Design review of the part built by this model. Coordinates are the model's own, in mm. Face numbers are marked on the shaded views. A direction names the side the tool comes from. Give positions to 0.01 mm unless a question says otherwise; leave off trailing zeros. Write each loop counter-clockwise with the first axis right and the second up, starting at its lowest first coordinate (ties: lowest second). Pieces come first, ordered by that corner, then holes. Notation, with made-up numbers: (-32, 68.25) -> (0, 68.25) arc R20 ccw to (0, 93.25) -> close; hole circle Ø11 at (-38.5, 69.5). An arc over 180 degrees is marked (long way). Answer as a JSON object with one key per item and string values.
```python
from build123d import *

# Parameters (mm, degrees)
SKETCH1_W                                      = 135
SKETCH1_H                                      = 103
BOSS_EXTRUDE1_DEPTH                            = 13
SKETCH2_W                                      = 127.02
SKETCH2_H                                      = 95.02
CUT_EXTRUDE1_DEPTH                             = 10
SKETCH3_R                                      = 6
CUT_EXTRUDE2_DEPTH                             = 2
FILLET1_R                                      = 1
FILLET1_OF_MIRROR1_R                           = 1
SKETCH4_R                                      = 6
CUT_EXTRUDE3_DEPTH                             = 2
FILLET2_R                                      = 1
FILLET2_OF_MIRROR2_R                           = 1
SKETCH5_W                                      = 31
SKETCH5_H                                      = 2.5
CUT_EXTRUDE4_DEPTH                             = 5
SKETCH6_W                                      = 135
SKETCH6_H                                      = 103
CUT_EXTRUDE5_DEPTH                             = 3.5
SKETCH7_W                                      = 33
SKETCH7_H                                      = 12
CUT_EXTRUDE6_DEPTH                             = 5
SKETCH8_OUTSIDE_W                              = 171.014
SKETCH8_OUTSIDE_H                              = 139.014
SKETCH8_OUTSIDE_W_2                            = 131
SKETCH8_OUTSIDE_H_2                            = 99
CUT_AROUND_SIDE_FOR_FRICTION_FITTING_COV_DEPTH = 1.5
SKETCH9_W                                      = 15
SKETCH9_H                                      = 2
CUT_EXTRUDE8_DEPTH                             = 1.5
FILLET3_R                                      = 5
FILLET4_R                                      = 2
SKETCH14_W                                     = 8.2
SKETCH14_H                                     = 1.5
CUT_EXTRUDE13_DEPTH                            = 4
SKETCH16_W                                     = 8.2
SKETCH16_H                                     = 1.5
CUT_EXTRUDE14_DEPTH                            = 4
SKETCH17_W                                     = 1.99
SKETCH17_H                                     = 1.5
CUT_EXTRUDE15_DEPTH                            = 9.3
CUT_EXTRUDE15_DEPTH_BACK                       = 1.1
SKETCH18_W                                     = 1.99
SKETCH18_H                                     = 1.5
CUT_EXTRUDE16_DEPTH                            = 9.3
CUT_EXTRUDE16_DEPTH_BACK                       = 1.1
SKETCH19_W                                     = 10.4
SKETCH19_H                                     = 4.692472087
SKETCH19_W_2                                   = 10.469305177
SKETCH19_H_2                                   = 5.245813632
CUT_EXTRUDE17_DEPTH                            = 3.1
SKETCH23_W                                     = 3.99
SKETCH23_H                                     = 3.1
BOSS_EXTRUDE2_DEPTH                            = 0.069305
CUT_EXTRUDE20_DEPTH                            = 0.2
CUT_EXTRUDE21_DEPTH                            = 0.4
CUT_EXTRUDE22_DEPTH                            = 0.3
CUT_EXTRUDE23_DEPTH                            = 0.3
SCALE1_SCALE                                   = 1.015


with BuildPart() as part:
    # Sketch1 → Boss-Extrude1 (new body)
    with BuildSketch(Plane(origin=(0, 0, 0), x_dir=(1, 0, 0), z_dir=(0, 1, 0))):
        Rectangle(SKETCH1_W, SKETCH1_H)
    extrude(amount=BOSS_EXTRUDE1_DEPTH)

    # Sketch2 → Cut-Extrude1 (cut)
    with BuildSketch(Plane(origin=(0, 13, 0), x_dir=(1, 0, 0), z_dir=(0, 1, 0))):
        Rectangle(SKETCH2_W, SKETCH2_H)
    extrude(amount=-CUT_EXTRUDE1_DEPTH, mode=Mode.SUBTRACT)

    # Sketch3 → Cut-Extrude2 (cut)
    with BuildSketch(Plane(origin=(0, 3, 0), x_dir=(1, 0, 0), z_dir=(0, 1, 0))):
        with Locations((-52.51, -36.51)):
            Circle(SKETCH3_R)
    cut_extrude2 = extrude(amount=-CUT_EXTRUDE2_DEPTH, mode=Mode.SUBTRACT)

    # Fillet1
    fillet1_edges = [part.edges().sort_by_distance(p)[0] for p in [
        (-58.51, 1, 36.51),
    ]]
    fillet(fillet1_edges, radius=FILLET1_R)

    # Mirror1: Cut-Extrude2 across plane
    add(cut_extrude2.mirror(Plane(origin=(0, 0, 0), x_dir=(0, 0, 1), z_dir=(1, 0, 0))), mode=Mode.SUBTRACT)

    # Fillet1 of Mirror1
    fillet1_of_mirror1_edges = [part.edges().sort_by_distance(p)[0] for p in [
        (58.51, 1, 36.51),
    ]]
    fillet(fillet1_of_mirror1_edges, radius=FILLET1_OF_MIRROR1_R)

    # Sketch4 → Cut-Extrude3 (cut)
    with BuildSketch(Plane(origin=(0, 3, 0), x_dir=(1, 0, 0), z_dir=(0, 1, 0))):
        with Locations((-44.51, 36.51)):
            Circle(SKETCH4_R)
    cut_extrude3 = extrude(amount=-CUT_EXTRUDE3_DEPTH, mode=Mode.SUBTRACT)

    # Fillet2
    fillet2_edges = [part.edges().sort_by_distance(p)[0] for p in [
        (-50.51, 1, -36.51),
    ]]
    fillet(fillet2_edges, radius=FILLET2_R)

    # Mirror2: Cut-Extrude3 across plane
    add(cut_extrude3.mirror(Plane(origin=(0, 0, 0), x_dir=(0, 0, 1), z_dir=(1, 0, 0))), mode=Mode.SUBTRACT)

    # Fillet2 of Mirror2
    fillet2_of_mirror2_edges = [part.edges().sort_by_distance(p)[0] for p in [
        (50.51, 1, -36.51),
    ]]
    fillet(fillet2_of_mirror2_edges, radius=FILLET2_OF_MIRROR2_R)

    # Sketch5 → Cut-Extrude4 (cut)
    with BuildSketch(Plane.ZY.offset(67.5)):
        with Locations((-30.05, 9.25)):
            Rectangle(SKETCH5_W, SKETCH5_H)
    extrude(amount=-CUT_EXTRUDE4_DEPTH, mode=Mode.SUBTRACT)

    # Sketch6 → Cut-Extrude5 (cut)
    with BuildSketch(Plane(origin=(0, 13, 0), x_dir=(1, 0, 0), z_dir=(0, 1, 0))):
        Rectangle(SKETCH6_W, SKETCH6_H)
    extrude(amount=-CUT_EXTRUDE5_DEPTH, mode=Mode.SUBTRACT)

    # Sketch7 → Cut-Extrude6 (cut)
    with BuildSketch(Plane(origin=(67.5, 0, 0), x_dir=(0, 0, -1), z_dir=(1, 0, 0))):
        with Locations((-3, 14)):
            Rectangle(SKETCH7_W, SKETCH7_H)
    extrude(amount=-CUT_EXTRUDE6_DEPTH, mode=Mode.SUBTRACT)

    # Sketch8 outside → Cut Around side for friction fitting cover (cut)
    with BuildSketch(Plane(origin=(0, 9.5, 0), x_dir=(1, 0, 0), z_dir=(0, 1, 0))):
        Rectangle(SKETCH8_OUTSIDE_W, SKETCH8_OUTSIDE_H)
        Rectangle(SKETCH8_OUTSIDE_W_2, SKETCH8_OUTSIDE_H_2, mode=Mode.SUBTRACT)
    extrude(amount=-CUT_AROUND_SIDE_FOR_FRICTION_FITTING_COV_DEPTH, mode=Mode.SUBTRACT)

    # Sketch9 → Cut-Extrude8 (cut)
    with BuildSketch(Plane(origin=(0, 8, 0), x_dir=(1, 0, 0), z_dir=(0, 1, 0))):
        with Locations((0, -50.5)):
            Rectangle(SKETCH9_W, SKETCH9_H)
    extrude(amount=-CUT_EXTRUDE8_DEPTH, mode=Mode.SUBTRACT)

    # Fillet3
    fillet3_edges = [part.edges().sort_by_distance(p)[0] for p in [
        (67.5, 4, 51.5),
        (-67.5, 4, 51.5),
        (-67.5, 4, -51.5),
        (67.5, 4, -51.5),
    ]]
    fillet(fillet3_edges, radius=FILLET3_R)

    # Fillet4
    fillet4_edges = [part.edges().sort_by_distance(p)[0] for p in [
        (67.5, 0, 0),
        (0, 0, 51.5),
        (-67.5, 0, 0),
        (0, 0, -51.5),
        (-66.035533906, 0, 50.035533906),
        (-66.035533906, 0, -50.035533906),
        (66.035533906, 0, -50.035533906),
        (66.035533906, 0, 50.035533906),
    ]]
    fillet(fillet4_edges, radius=FILLET4_R)

    # Sketch14 → Cut-Extrude13 (cut)
    with BuildSketch(Plane.XY.offset(49.5)):
        with Locations((-56.5, 8.75)):
            Rectangle(SKETCH14_W, SKETCH14_H)
    extrude(amount=-CUT_EXTRUDE13_DEPTH, mode=Mode.SUBTRACT)

    # Sketch16 → Cut-Extrude14 (cut)
    with BuildSketch(Plane.XY.offset(49.5)):
        with Locations((-41.5, 8.75)):
            Rectangle(SKETCH16_W, SKETCH16_H)
    extrude(amount=-CUT_EXTRUDE14_DEPTH, mode=Mode.SUBTRACT)

    # Sketch17 → Cut-Extrude15 (cut, two sides)
    with BuildSketch(Plane(origin=(-60.6, 0, 0), x_dir=(0, 0, -1), z_dir=(1, 0, 0))) as cut_extrude15_sk:
        with Locations((-48.505, 8.75)):
            Rectangle(SKETCH17_W, SKETCH17_H)
    extrude(amount=CUT_EXTRUDE15_DEPTH, mode=Mode.SUBTRACT)
    extrude(cut_extrude15_sk.sketch, amount=-CUT_EXTRUDE15_DEPTH_BACK, mode=Mode.SUBTRACT)

    # Sketch18 → Cut-Extrude16 (cut, two sides)
    with BuildSketch(Plane(origin=(-45.6, 0, 0), x_dir=(0, 0, -1), z_dir=(1, 0, 0))) as cut_extrude16_sk:
        with Locations((-48.505, 8.75)):
            Rectangle(SKETCH18_W, SKETCH18_H)
    extrude(amount=CUT_EXTRUDE16_DEPTH, mode=Mode.SUBTRACT)
    extrude(cut_extrude16_sk.sketch, amount=-CUT_EXTRUDE16_DEPTH_BACK, mode=Mode.SUBTRACT)

    # Sketch19 → Cut-Extrude17 (cut)
    with BuildSketch(Plane(origin=(0, 8, 0), x_dir=(1, 0, 0), z_dir=(0, 1, 0))):
        with Locations((-56.5, -49.856236044)):
            Rectangle(SKETCH19_W, SKETCH19_H)
        with Locations((-41.465347412, -50.132906816)):
            Rectangle(SKETCH19_W_2, SKETCH19_H_2)
    extrude(amount=-CUT_EXTRUDE17_DEPTH, mode=Mode.SUBTRACT)

    # Sketch23 → Boss-Extrude2 (add)
    with BuildSketch(Plane.ZY.offset(36.230694823)):
        with Locations((49.505, 6.45)):
            Rectangle(SKETCH23_W, SKETCH23_H)
    extrude(amount=BOSS_EXTRUDE2_DEPTH)

    # Sketch24 → Cut-Extrude20 (cut)
    with BuildSketch(Plane.ZY.offset(36.3)):
        Polygon((47.51, 4.9), (47.51, 9.5), (49.5, 9.5), (49.5, 8), (51.5, 8), (51.5, 4.9), align=None)
    extrude(amount=-CUT_EXTRUDE20_DEPTH, mode=Mode.SUBTRACT)

    # Sketch25 → Cut-Extrude21 (cut)
    with BuildSketch(Plane(origin=(-46.7, 0, 0), x_dir=(0, 0, -1), z_dir=(1, 0, 0))):
        Polygon((-51.5, 4.9), (-47.51, 4.9), (-47.51, 9.5), (-49.5, 9.5), (-49.5, 8), (-51.5, 8), align=None)
    extrude(amount=-CUT_EXTRUDE21_DEPTH, mode=Mode.SUBTRACT)

    # Sketch26 → Cut-Extrude22 (cut)
    with BuildSketch(Plane.ZY.offset(51.3)):
        Polygon((47.51, 9.5), (47.51, 4.9), (51.5, 4.9), (51.5, 8), (49.5, 8), (49.5, 9.5), align=None)
    extrude(amount=-CUT_EXTRUDE22_DEPTH, mode=Mode.SUBTRACT)

    # Sketch27 → Cut-Extrude23 (cut)
    with BuildSketch(Plane(origin=(-61.7, 0, 0), x_dir=(0, 0, -1), z_dir=(1, 0, 0))):
        Polygon((-51.5, 4.9), (-47.51, 4.9), (-47.51, 9.5), (-49.5, 9.5), (-49.5, 8), (-51.5, 8), align=None)
    extrude(amount=-CUT_EXTRUDE23_DEPTH, mode=Mode.SUBTRACT)


with BuildPart() as part_1:
    # Scale1: scaled about (0, 0, 0)
    add(part.part.scale(SCALE1_SCALE))


solid = part_1.part
```
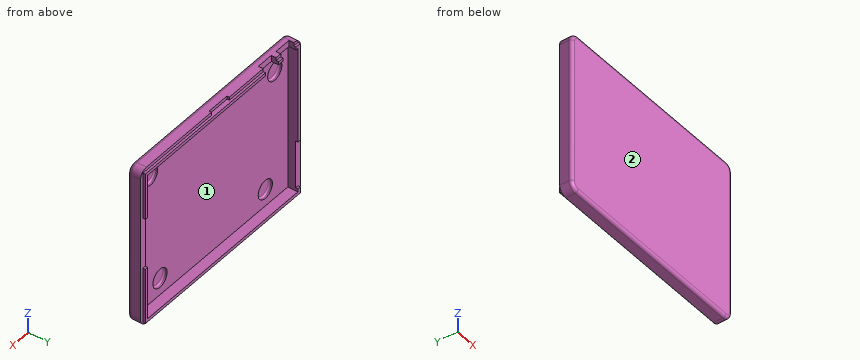
(1) Clearance check with flat-ended pins moving along their axes: pin 1 (1 mm diameter, centred on x = -25, z = 25, fed in from +Y) (3 decimals); pin 2 (1.7 mm diameter, centred on y = 9.5, z = -47.5, fed in from -X); pin 3 (5 mm diameter, centred on x = -47.5, z = -37, fed in from +Y) (3 decimals). State where each tip first meets the part, or that it passes through.
Here are the results:
{"pin 1": "stops at y = 3.045", "pin 2": "stops at x = -66.48", "pin 3": "stops at y = 1.015"}
(2) For the marked faces 1 and 2, list the 3-axis set-ups (+Z, -Z, +X, -X, +Y, -Y) from which the entire face can be reached by the end or side of a thin tool; tool diameter is ignored.
Here are the results:
{"face 1": "+Y", "face 2": "+Z, -Z, +X, -X, -Y"}
(3) We need section B-B, the plane x = 14. State the section outline as (y, z) points (1 decimal), then the cut area to 3 significant figures.
Here are the results:
{"outline": "(0, -50.2) arc R2 ccw to (2, -52.3) -> (8.1, -52.3) -> (8.1, -50.2) -> (9.6, -50.2) -> (9.6, -48.2) -> (3, -48.2) -> (3, 48.2) -> (9.6, 48.2) -> (9.6, 50.2) -> (8.1, 50.2) -> (8.1, 52.3) -> (2, 52.3) arc R2 ccw to (0, 50.2) -> close", "area": "364 mm²"}
(4) We need section A-A, the plane z = -22. State the section outline as (x, y) points (1 decimal).
Here are the results:
{"outline": "(-68.5, 2) arc R2 ccw to (-66.5, 0) -> (66.5, 0) arc R2 ccw to (68.5, 2) -> (68.5, 8.1) -> (66.5, 8.1) -> (66.5, 9.6) -> (64.5, 9.6) -> (64.5, 3) -> (-64.5, 3) -> (-64.5, 8.1) -> (-68.5, 8.1) -> close"}
(5) For line 1 along X through (y, z) = (6.5, 33); line 2 along Z through (x, y) = (0.5, 7.5); line 3 along Z through (x, y) = (-49.5, 9), list the stretches that pass through material, from the lowest coordinate up.
Here are the results:
{"line 1": "x = -68.51 to -64.46, 64.46 to 68.51", "line 2": "z = -52.27 to -48.22, 48.22 to 50.24", "line 3": "z = -50.24 to -48.22, 48.22 to 50.24"}
(6) We need section C-C, the plane x = -1. State the section outline as (y, z) points (1 decimal), then the cut area to 3 significant figures.
Here are the results:
{"outline": "(0, -50.2) arc R2 ccw to (2, -52.3) -> (8.1, -52.3) -> (8.1, -50.2) -> (9.6, -50.2) -> (9.6, -48.2) -> (3, -48.2) -> (3, 48.2) -> (9.6, 48.2) -> (9.6, 50.2) -> (6.6, 50.2) -> (6.6, 52.3) -> (2, 52.3) arc R2 ccw to (0, 50.2) -> close", "area": "361 mm²"}
